Geometry: final body of the model. Coordinates: model frame, mm. A direction names the side the tool comes from. Round coordinates to 2 decimals unless told otherwise and drop trailing zeros. Loops run counter-clockwise (first coordinate to the right, second up) from the corner with the lowest first, then second, coordinate; pieces in that order, holes last. Notation, with made-up numbers: M 72.25,22.5 L 116.25,22.5 A29 cw 116.25,49.5 Z; hole C 49.25,5 d5. An arc over 180 degrees is marked long. Write each question's results on one line, items separated by ' | '.
Autodesk Inventor part; units mm, degrees
ref_plane "YZ Plane" through (0, 0, 0) normal (1, 0, 0) x (0, 1, 0)
ref_plane "XZ Plane" through (0, 0, 0) normal (0, 1, 0) x (-1, 0, 0)
ref_plane "XY Plane" through (0, 0, 0) normal (0, 0, 1) x (1, 0, 0)
sketch "Szkic1" plane through (0, 0, 0) normal (0, 1, 0) x (-1, 0, 0)
  line L0 (20, 25) -> (-20, 25)
  line L1 (-20, 25) -> (-20, -25)
  line L2 (-20, -25) -> (20, -25)
  line L3 (20, -25) -> (20, 25)
  line L4 (20, 25) -> (-20, -25) construction
  line L5 (-20, 25) -> (20, -25) construction
  line L6 (26, 31) -> (14, 31)
  line L7 (14, 31) -> (14, 19)
  line L8 (14, 19) -> (26, 19)
  line L9 (26, 19) -> (26, 31)
  line L10 (26, 31) -> (14, 19) construction
  line L11 (14, 31) -> (26, 19) construction
  line L12 (26, -19) -> (14, -19)
  line L13 (14, -19) -> (14, -31)
  line L14 (14, -31) -> (26, -31)
  line L15 (26, -31) -> (26, -19)
  line L16 (26, -19) -> (14, -31) construction
  line L17 (14, -19) -> (26, -31) construction
  line L18 (-14, 31) -> (-26, 31)
  line L19 (-26, 31) -> (-26, 19)
  line L20 (-26, 19) -> (-14, 19)
  line L21 (-14, 19) -> (-14, 31)
  line L22 (-14, 31) -> (-26, 19) construction
  line L23 (-26, 31) -> (-14, 19) construction
  line L24 (-14, -19) -> (-26, -19)
  line L25 (-26, -19) -> (-26, -31)
  line L26 (-26, -31) -> (-14, -31)
  line L27 (-14, -31) -> (-14, -19)
  line L28 (-14, -19) -> (-26, -31) construction
  line L29 (-26, -19) -> (-14, -31) construction
  point P0 (0, 0)
  point P1 (20, 19)
  point P2 (-14, -25)
  point P3 (-26, -25)
  point P4 (-20, -19)
  point P5 (-20, -31)
  dimension "d0" = 50
  dimension "d1" = 40
  dimension "d2" = 12
  dimension "d3" = 12
  dimension "d4" = 12
  dimension "d5" = 12
  dimension "d6" = 12
  dimension "d7" = 12
  dimension "d8" = 12
  dimension "d9" = 12
extrude "Wyciągnięcie proste1" add sketch "Szkic1" along normal blind 30 contours L3 L8 L7 L0 | L0 L7 L6 L9 L8 L3 | L21 L20 L1 L0 | L0 L1 L20 L19 L18 L21 | L12 L15 L14 L13 L2 L3 | L3 L2 L13 L12 | L24 L27 L2 L1 | L1 L2 L27 L26 L25 L24
sketch "Szkic2" plane through (0, 30, 0) normal (0, 1, 0) x (1, 0, 0)
  line L0 (-26, -19) -> (-26, -31)
  line L1 (26, 31) -> (14, 31)
  line L2 (-26, -31) -> (26, -31)
  line L3 (26, -31) -> (26, 31)
  line L4 (26, 31) -> (-26, 31)
  line L5 (-26, 31) -> (-26, -31)
  point P0 (0, 0)
extrude "Wyciągnięcie proste2" add sketch "Szkic2" along normal blind 4
sketch "Szkic3" plane through (0, 0, 0) normal (0, -1, 0) x (1, 0, 0)
  circle A0 centre (-20, 25) radius 2.5
  circle A1 centre (20, 25) radius 2.5
  circle A2 centre (-20, -25) radius 2.5
  circle A3 centre (20, -25) radius 2.5
  line L0 (-14, 19) -> (-26, 19)
  line L1 (26, 19) -> (14, 19)
  line L2 (-26, -19) -> (-14, -19)
  line L3 (14, -19) -> (26, -19)
  line L4 (14, -31) -> (14, -19)
  line L5 (-26, -31) -> (-26, -19)
  line L6 (-26, 19) -> (-26, 31)
  line L7 (14, 19) -> (14, 31)
  point P0 (0, 0)
  point P1 (-20, 19)
  point P2 (-20, -19)
  point P3 (-26, -25)
  dimension "d14" = 5
  dimension "d15" = 6
  dimension "d16" = 6
  dimension "d17" = 6
  dimension "d18" = 6
  dimension "d19" = 6
  dimension "d20" = 6
  dimension "d21" = 6
  dimension "d22" = 6
  dimension "d23" = 5
  dimension "d24" = 5
  dimension "d25" = 5
extrude "Wyciągnięcie proste3" cut sketch "Szkic3" against normal blind 34
sketch "Szkic4" plane through (0, 34, 0) normal (0, 1, 0) x (1, 0, 0)
  circle A0 centre (20, 25) radius 2.5
  circle A1 centre (20, 25) radius 4
  circle A2 centre (20, -25) radius 2.5
  circle A3 centre (20, -25) radius 4
  circle A4 centre (-20, -25) radius 2.5
  circle A5 centre (-20, -25) radius 4
  circle A6 centre (-20, 25) radius 2.5
  circle A7 centre (-20, 25) radius 4
  point P0 (0, 0)
  dimension "d28" = 8
  dimension "d29" = 8
  dimension "d30" = 8
  dimension "d31" = 8
extrude "Wyciągnięcie proste4" cut sketch "Szkic4" against normal blind 22
sketch "Szkic5" plane through (0, 34, 0) normal (0, 1, 0) x (1, 0, 0)
  line L0 (14.5, 8.5) -> (14.5, -8.5) construction
  line L1 (13, 8.5) -> (13, -8.5)
  line L2 (16, -8.5) -> (16, 8.5)
  arc A0 (16, 8.5) -> (13, 8.5) centre (14.5, 8.5) ccw
  arc A1 (13, -8.5) -> (16, -8.5) centre (14.5, -8.5) ccw
  line L3 (8.5, 19.5) -> (-8.5, 19.5) construction
  line L4 (8.5, 21) -> (-8.5, 21)
  line L5 (-8.5, 18) -> (8.5, 18)
  arc A2 (8.5, 18) -> (8.5, 21) centre (8.5, 19.5) ccw
  arc A3 (-8.5, 21) -> (-8.5, 18) centre (-8.5, 19.5) ccw
  line L6 (-14.5, 8.5) -> (-14.5, -8.5) construction
  line L7 (-16, 8.5) -> (-16, -8.5)
  line L8 (-13, -8.5) -> (-13, 8.5)
  arc A4 (-13, 8.5) -> (-16, 8.5) centre (-14.5, 8.5) ccw
  arc A5 (-16, -8.5) -> (-13, -8.5) centre (-14.5, -8.5) ccw
  line L9 (-8.5, -19.5) -> (8.5, -19.5) construction
  line L10 (-8.5, -21) -> (8.5, -21)
  line L11 (8.5, -18) -> (-8.5, -18)
  arc A6 (-8.5, -18) -> (-8.5, -21) centre (-8.5, -19.5) ccw
  arc A7 (8.5, -21) -> (8.5, -18) centre (8.5, -19.5) ccw
  line L12 (26, 31) -> (-26, 31)
  line L13 (26, -31) -> (26, 31)
  line L14 (-26, -31) -> (26, -31)
  line L15 (-26, 31) -> (-26, -31)
  point P0 (0, 0)
  point P1 (14.5, 0)
  point P2 (0, 19.5)
  point P3 (-14.5, 0)
  point P4 (0, -19.5)
  point P5 (-16, 0)
  point P6 (-26, 0)
  point P7 (10, 19.5)
  point P8 (-10, 19.5)
  point P9 (10, -19.5)
  point P10 (-10, -19.5)
  point P11 (14.5, -10)
  point P12 (14.5, 10)
  point P13 (-14.5, -10)
  point P14 (-14.5, 10)
  dimension "d34" = 10
  dimension "d35" = 10
  dimension "d36" = 10
  dimension "d37" = 3
  dimension "d38" = 10
  dimension "d39" = 20
  dimension "d40" = 20
  dimension "d41" = 20
  dimension "d42" = 20
  dimension "d43" = 3
  dimension "d44" = 3
  dimension "d45" = 3
  dimension "d46" = 31
  dimension "d47" = 31
  dimension "d48" = 26
  dimension "d49" = 26
extrude "Wyciągnięcie proste5" cut sketch "Szkic5" against normal blind 22 contours A0 L2 A1 L1 | A2 L5 A3 L4 | A4 L8 A5 L7 | A6 L11 A7 L10
properties part number "wires_keeper_Drukowanie 3D"
1. Section B-B (x = 20). Output: boundary loops of the cut face in (y, z).
Answer key:
outline: M 0,-31 L 34,-31 L 34,-29 L 12,-29 L 12,-27.5 L 0,-27.5 Z; M 0,-22.5 L 12,-22.5 L 12,-21 L 34,-21 L 34,21 L 12,21 L 12,22.5 L 0,22.5 L 0,19 L 30,19 L 30,-19 L 0,-19 Z; M 0,27.5 L 12,27.5 L 12,29 L 34,29 L 34,31 L 0,31 Z
2. Ray query, probe 1 along X at (y, z) = (8.5, -25); probe 2 along X at (y, z) = (24, -25); probe 3 along X at (y, z) = (30.5, 3). Return the intervals inside material, ascending.
Answer key:
probe 1: x = -26 to -22.5, -17.5 to -14, 14 to 17.5, 22.5 to 26 | probe 2: x = -26 to -24, -16 to -14, 14 to 16, 24 to 26 | probe 3: x = -26 to -16, -13 to 13, 16 to 26
3. Section A-A (y = 10.5). Output: boundary loops of the cut face in (x, z).
Answer key:
outline: M -26,-31 L -14,-31 L -14,-19 L -26,-19 Z; M -26,19 L -14,19 L -14,31 L -26,31 Z; M 14,-31 L 26,-31 L 26,-19 L 14,-19 Z; M 14,19 L 26,19 L 26,31 L 14,31 Z; hole C -20,-25 d5; hole C -20,25 d5; hole C 20,-25 d5; hole C 20,25 d5
4. Pin query (flat end, axial travel): P1, Ø2, axis at x = -10, z = -19, coming from the -Y side. Return the tip coordinate at first contact, or that it passes through.
Answer key:
P1: stops at y = 30
5. Access query for faces 1 (the face through (16, 32, 0)), 2 (the face through (-20, 15, -19)), 3 (the face through (19.479, 23.154, 21.034)), 4 (the face through (14, 15, -25)). Directions: +Z, -Z, +X, -X, +Y, -Y. A direction counts if a zero-diameter tool reaches every point of the face in a straight line with its end or side. Return the directions, or none.
Answer key:
face 1: +Y, -Y | face 2: +X, -X, -Y | face 3: +Y | face 4: +Z, -Z, -Y
6. Section C-C (z = 25). Output: boundary loops of the cut face in (x, y).
Answer key:
outline: M -26,0 L -22.5,0 L -22.5,12 L -24,12 L -24,34 L -26,34 Z; M -17.5,0 L -14,0 L -14,30 L 14,30 L 14,0 L 17.5,0 L 17.5,12 L 16,12 L 16,34 L -16,34 L -16,12 L -17.5,12 Z; M 22.5,0 L 26,0 L 26,34 L 24,34 L 24,12 L 22.5,12 Z
7. Draft query along X for faces 5 (the face through (14.5, 32, -10)), 6 (the face through (-23, 0, 25)), 7 (the face through (-26, 32, 0)). Return one class per face: pulls with the +X half, pulls with the -X half, needs draft (parallel to the pull), parting line crosses it, or undercut.
Answer key:
face 5: undercut | face 6: needs draft | face 7: pulls with the -X half
8. Section D-D (y = 14.5). Output: boundary loops of the cut face in (x, z).
Answer key:
outline: M -26,-31 L -14,-31 L -14,-19 L -26,-19 Z; M -26,19 L -14,19 L -14,31 L -26,31 Z; M 14,-31 L 26,-31 L 26,-19 L 14,-19 Z; M 14,19 L 26,19 L 26,31 L 14,31 Z; hole C -20,-25 d8; hole C -20,25 d8; hole C 20,-25 d8; hole C 20,25 d8
